from build123d import *

# Parameters (mm, degrees)
SKETCH1_R           = 32.5
SKETCH1_R_2         = 2.5
BOSS_EXTRUDE1_DEPTH = 5
SKETCH2_R           = 10
BOSS_EXTRUDE2_DEPTH = 14.5
SKETCH3_R           = 3.1
CUT_EXTRUDE1_DEPTH  = 24.5
CUT_EXTRUDE3_START  = -14.5
CUT_EXTRUDE3_DEPTH  = 14.5
SKETCH8_R           = 1.5
CUT_EXTRUDE5_DEPTH  = 5
CHAMFER2_SIZE       = 0.5


with BuildPart() as part:
    # Sketch1 → Boss-Extrude1 (new body)
    with BuildSketch(Plane.XY):
        Circle(SKETCH1_R)
        with Locations((0, 20)):
            Circle(SKETCH1_R_2, mode=Mode.SUBTRACT)
        with Locations((-17.320508076, -10)):
            Circle(SKETCH1_R_2, mode=Mode.SUBTRACT)
        with Locations((17.320508076, -10)):
            Circle(SKETCH1_R_2, mode=Mode.SUBTRACT)
    extrude(amount=BOSS_EXTRUDE1_DEPTH)

    # Sketch2 → Boss-Extrude2 (add)
    with BuildSketch(Plane(origin=(0, 0, 0), x_dir=(-1, 0, 0), z_dir=(0, 0, -1))):
        with Locations(Location((0, 0, 0), (0, 0, 180))):
            Circle(SKETCH2_R)
    extrude(amount=BOSS_EXTRUDE2_DEPTH)

    # Sketch3 → Cut-Extrude1 (cut)
    with BuildSketch(Plane(origin=(0, 0, -14.5), x_dir=(-1, 0, 0), z_dir=(0, 0, -1))):
        Circle(SKETCH3_R)
    extrude(amount=-CUT_EXTRUDE1_DEPTH, mode=Mode.SUBTRACT)

    # Sketch7 → Cut-Extrude3 (cut)
    with BuildSketch(Plane(origin=(0, 0, -14.5), x_dir=(-1, 0, 0), z_dir=(0, 0, -1)).offset(CUT_EXTRUDE3_START)):
        with BuildLine():
            Line((0, 6.5), (-7.599342077, 6.5))
            ThreePointArc((-7.599342077, 6.5), (0, 10), (7.599342077, 6.5))
            Line((7.599342077, 6.5), (0, 6.5))
        make_face()
    extrude(amount=CUT_EXTRUDE3_DEPTH, mode=Mode.SUBTRACT)

    # Sketch8 → Cut-Extrude5 (cut)
    with BuildSketch(Plane(origin=(0, 6.5, 0), x_dir=(1, 0, 0), z_dir=(0, 1, 0))):
        with Locations(Location((0, 7.25, 0), (0, 0, 180))):
            Circle(SKETCH8_R)
    extrude(amount=-CUT_EXTRUDE5_DEPTH, mode=Mode.SUBTRACT)

    # Chamfer2
    chamfer2_edges = [part.edges().sort_by_distance(p)[0] for p in [
        (-32.5, 0, 0),
        (0, -10, -14.5),
        (0, -10, 0),
        (-32.5, 0, 5),
    ]]
    chamfer(chamfer2_edges, length=CHAMFER2_SIZE)


solid = part.part
Read the model definition and answer for the solid it produces. Units are mm, in the model's axes. A direction names the side the tool comes from. Round coordinates to 2 decimals unless told otherwise and drop trailing zeros. Write each loop counter-clockwise with the first axis right and the second up, starting at its lowest first coordinate (ties: lowest second). Pieces come first, ordered by that corner, then holes. Notation, with made-up numbers: (49.25, 68) - (58.25, 68) arc R16 cw to (58.25, 97) - close; hole circle Ø11 at (86.25, -21.5). An arc over 180 degrees is marked (long way). One line per question, with ' | ' between items. Start each with the question number.
1. Section D-D (z = -2.75) is taken. Determine the outline of the cut face in (x, y).
2. Section A-A (x = 0) is taken. Determine the outline of the cut face in (y, z), and give its area (3 significant figures).
3. Find the intervals of material crossed by probe 1 along Y at (x, z) = (0, 3.35); probe 2 along Y at (x, z) = (0, -4); probe 3 along Z at (x, y) = (0, 5.45), in increasing order. Write a range as [from, to].
4. For faces 4 (the face through (1.5, 4.6, -7.2)), 5 (the face through (-0.323, -10.13, -0.365)), 6 (the face through (-0.1, 6.5, -5.5)), determine the directions among +Z, -Z, +X, -X, +Y, -Y from which every point of the face is accessible in a straight line to the end or side of a thin tool.
5. For a pull along Y with two mould halves and no side action, classify faces 1 (the face through (0.672, -3.026, -4.886)), 2 (the face through (0, -10, -7)), 3 (the face through (-0.1, -3.4, -14.5)) as +Y half, -Y half, draft (parallel to the pull), parting line (faces both ways), or undercut.
6. Each of these flat-tipped pins is pushed along its axis until it touches: pin 1 (4 mm diameter, centred on y = -7.5, z = -7, fed in from -X); pin 2 (7 mm diameter, centred on x = 0, y = 0, fed in from +Z); pin 3 (4.5 mm diameter, centred on x = 17.32, y = -10, fed in from +Z); pin 4 (1 mm diameter, centred on x = 2, y = -20.5, fed in from -Z). Where does it stop, or does it pass through?
7. Section C-C (z = -7.25) is taken. Determine the outline of the cut face in (x, y), and give its area (3 significant figures).
8. Section B-B (y = 0) is taken. Determine the outline of the cut face in (x, z).
Filled in:
1) outline: (-7.6, 6.5) arc R10 ccw (long way) to (7.6, 6.5) - close; hole circle Ø6.2 at (0, 0)
2) outline: (-32.5, 0.5) - (-32, 0) - (-10.5, 0) - (-10, -0.5) - (-10, -14) - (-9.5, -14.5) - (-3.1, -14.5) - (-3.1, 5) - (-32, 5) - (-32.5, 4.5) - close; (3.1, -14.5) - (6.5, -14.5) - (6.5, -8.75) - (3.1, -8.75) - close; (3.1, -5.75) - (6.5, -5.75) - (6.5, 0) - (17.5, 0) - (17.5, 5) - (3.1, 5) - close; (22.5, 0) - (32, 0) - (32.5, 0.5) - (32.5, 4.5) - (32, 5) - (22.5, 5) - close | area: 408 mm²
3) probe 1: [-32.5, -3.1], [3.1, 17.5], [22.5, 32.5] | probe 2: [-10, -3.1], [3.1, 6.5] | probe 3: [-14.5, -8.75], [-5.75, 5]
4) face 4: +Y | face 5: -Z | face 6: -Z, +X, -X, +Y
5) face 1: undercut | face 2: parting line | face 3: draft
6) pin 1: x = -8.35 | pin 2: z = 5 | pin 3: through | pin 4: z = 0
7) outline: (-7.6, 6.5) arc R10 ccw (long way) to (7.6, 6.5) - (1.5, 6.5) - (1.5, 2.71) arc R3.1 cw (long way) to (-1.5, 2.71) - (-1.5, 6.5) - close | area: 236 mm²
8) outline: (-32.5, 0.5) - (-32, 0) - (-10.5, 0) - (-10, -0.5) - (-10, -14) - (-9.5, -14.5) - (-3.1, -14.5) - (-3.1, 5) - (-32, 5) - (-32.5, 4.5) - close; (3.1, -14.5) - (9.5, -14.5) - (10, -14) - (10, -0.5) - (10.5, 0) - (32, 0) - (32.5, 0.5) - (32.5, 4.5) - (32, 5) - (3.1, 5) - close
